Part model, mm, in its own coordinate system. Face numbers are marked on the shaded views. A direction names the side the tool comes from. Give positions to 0.01 mm unless a question says otherwise; leave off trailing zeros. Order: outer loops, then holes, each group sorted by start corner. A loop starts at its lowest first (then second) coordinate and runs counter-clockwise, first axis right, second up.
1. Probe line 1 (Y direction, x = 0, z = 3); line 2 (Z direction, x = 4, y = 12); line 3 (X direction, y = 1.25, z = 3.2). List the from-to ranges inside material, lowest first.
2. Slice it at C-C on x = 0. List the corners of the cut face in (y, z).
3. Which spindle directions (+Z, -Z, +X, -X, +Y, -Y) get a long thin tool onto all of the face, cutting with end or side? Do the marked faces 1 and 2. Say none if no direction does.
4. Slice it at A-A on y = 20. List the corners of the cut face in (x, z) (3 decimals).
5. Mould opens along X. For the marked faces 3, 4, 5 and 6 say: +X half, -X half, draft (parallel to the pull), parting line (faces both ways), or undercut.
6. Slice it at B-B on x = 4. List the corners of the cut face in (y, z), and give its area (3 significant figures).
7. Drop flat-ended pins along their axis: pin 1 Ø1.9 at (x, y) = (0, 20) entering from +Z; pin 2 Ø3.5 at (x, y) = (0, 2.5) entering from +Z. Give the stop position or say it passes through.
8. Slice it at D-D on z = 1.3. List the corners of the cut face in (x, y).
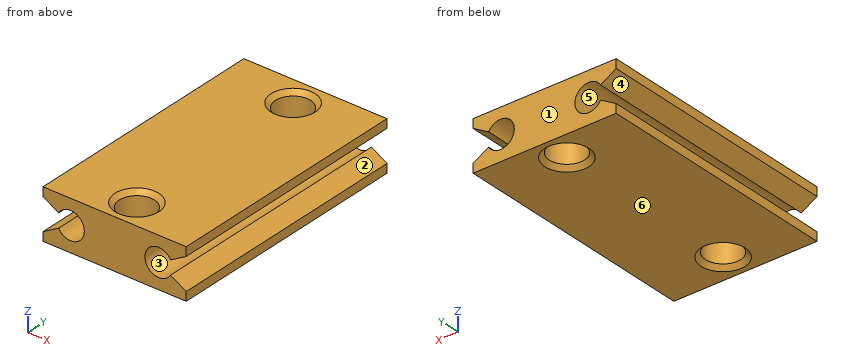
from build123d import *

# Parameters (mm, degrees)
BASE_SKETCH_W                 = 13
BASE_SKETCH_H                 = 4.5
BLOCK_SIZE_DEPTH              = 22.5
M3_CLEARANCE_HOLE1_AT_2_COUNT = 2
M3_CLEARANCE_HOLE1_AT_2_PITCH = 17.5
M3X0_5_TAPPED_HOLE1_D         = 2.5
SIDE_CUTS_DEPTH               = 23.5


with BuildPart() as part:
    # Base Sketch → Block Size (new body)
    with BuildSketch(Plane(origin=(0, 0, 0), x_dir=(1, 0, 0), z_dir=(0, 1, 0))):
        with Locations((0, -2.25)):
            Rectangle(BASE_SKETCH_W, BASE_SKETCH_H)
    extrude(amount=BLOCK_SIZE_DEPTH)

    # Sketch3 → M3 Clearance Hole1 (revolve, cut)
    with BuildSketch(Plane(origin=(0, 20, 0), x_dir=(0, 1, 0), z_dir=(1, 0, 0))):
        Polygon((0, 0), (0, 4.5), (2, 4.5), (1.6, 4.1), (1.6, 0.4), (2, 0), align=None)
    m3_clearance_hole1 = revolve(axis=Axis((0, 20, -6.35), (0, 0, 1)), mode=Mode.SUBTRACT)

    # M3 Clearance Hole1 at 2: M3 Clearance Hole1 ×2
    with Locations(*[(0, -i * M3_CLEARANCE_HOLE1_AT_2_PITCH, 0) for i in range(1, M3_CLEARANCE_HOLE1_AT_2_COUNT)]):
        add(m3_clearance_hole1, mode=Mode.SUBTRACT)

    # M3x0.5 Tapped Hole1 (through all)
    with Locations(Plane.XZ):
        with Locations((-3.999999936, 2.25), (3.999999936, 2.25)):
            Hole(M3X0_5_TAPPED_HOLE1_D / 2)

    # Sketch6 → Side Cuts (cut, through all)
    with BuildSketch(Plane(origin=(0, 0, 0), x_dir=(1, 0, 0), z_dir=(0, 1, 0))):
        Polygon((-6.5, -0.80662429), (-3.999999936, -2.25), (-6.5, -3.69337571), align=None)
        Polygon((3.999999936, -2.25), (6.5, -0.80662429), (6.5, -3.69337571), align=None)
    extrude(amount=SIDE_CUTS_DEPTH, mode=Mode.SUBTRACT)


solid = part.part
Data:
1. line 1: y = 0 to 0.9, 4.1 to 18.4, 21.6 to 22.5
1. line 2: z = 0 to 1, 3.5 to 4.5
1. line 3: x = -5.65 to -4.81, -3.19 to -1, 1 to 3.19, 4.81 to 5.65
2. outline: (0, 0) - (0.5, 0) - (0.9, 0.4) - (0.9, 4.1) - (0.5, 4.5) - (0, 4.5) - close; (4.1, 0.4) - (4.5, 0) - (18, 0) - (18.4, 0.4) - (18.4, 4.1) - (18, 4.5) - (4.5, 4.5) - (4.1, 4.1) - close; (21.6, 0.4) - (22, 0) - (22.5, 0) - (22.5, 4.5) - (22, 4.5) - (21.6, 4.1) - close
3. face 1: +Z, -Z, +X, -X, +Y
3. face 2: +X, +Y, -Y
4. outline: (-6.5, 0) - (-2, 0) - (-1.6, 0.4) - (-1.6, 4.1) - (-2, 4.5) - (-6.5, 4.5) - (-6.5, 3.693) - (-5.083, 2.875) arc R1.25 cw (long way) to (-5.083, 1.625) - (-6.5, 0.807) - close; (1.6, 0.4) - (2, 0) - (6.5, 0) - (6.5, 0.807) - (5.083, 1.625) arc R1.25 cw (long way) to (5.083, 2.875) - (6.5, 3.693) - (6.5, 4.5) - (2, 4.5) - (1.6, 4.1) - close
5. face 3: undercut
5. face 4: -X half
5. face 5: undercut
5. face 6: draft
6. outline: (0, 0) - (22.5, 0) - (22.5, 1) - (0, 1) - close; (0, 3.5) - (22.5, 3.5) - (22.5, 4.5) - (0, 4.5) - close
6. area: 45.0 mm2
7. pin 1: passes through
7. pin 2: stops at z = 4.25
8. outline: (-5.65, 0) - (-4.81, 0) - (-4.81, 22.5) - (-5.65, 22.5) - close; (-3.19, 0) - (3.19, 0) - (3.19, 22.5) - (-3.19, 22.5) - close; (4.81, 0) - (5.65, 0) - (5.65, 22.5) - (4.81, 22.5) - close; hole circle Ø3.2 at (0, 2.5); hole circle Ø3.2 at (0, 20)
